Here's how the part is built. I have some questions about the finished solid (model axes, mm). A direction names the side the tool comes from. Coordinates: 2 decimals unless noted, no trailing zeros. Write each loop counter-clockwise with the first axis right and the second up, starting at its lowest first coordinate (ties: lowest second). Pieces come first, ordered by that corner, then holes.
from build123d import *

# Parameters (mm, degrees)
F1_DEPTH    = 5.5
F2_DEPTH    = 15
F3_T1_DEPTH = 64.5730638659
F3_T3_DEPTH = 54.5730638659


# Not quite as in the source:
# - a fillet or chamfer that OpenCascade refuses, or shapes differently, is made with other operations: its cross-section is extruded or revolved along the edge and cut away or added


with BuildPart() as f1:
    # F0 (on Right) → F1 (new body, symmetric)
    with BuildSketch(Plane.YZ):
        Polygon((-11, 0), (0, 0), (0, 5), (-11, 5), (-11, 11), (-15, 11), (-15, 0), align=None)
    extrude(amount=F1_DEPTH, both=True)

    # F0 (on Right) → F2 (join, symmetric)
    with BuildSketch(Plane.YZ):
        Polygon((-15, 15), (-15, 11), (-11, 11), (25, 11), (25, 15), align=None)
    extrude(amount=F2_DEPTH, both=True)

    # F3: chamfer of 4 x 4.7670143704 on 3 edges, made by hand

    # F3_s2 → F3_t1 (cut)
    with BuildSketch(Plane.XZ.offset(-37.2865319329)):
        Polygon((15, 10.2329856296), (11, 15), (15, 15), align=None)
        Polygon((-15, 10.2329856296), (-11, 15), (-15, 15), align=None)
    extrude(amount=F3_T1_DEPTH, mode=Mode.SUBTRACT)

    # F3_s4 → F3_t3 (cut)
    with BuildSketch(Plane.YZ.offset(-27.2865319329)):
        Polygon((21, 15), (25, 10.2329856296), (25, 15), align=None)
    extrude(amount=F3_T3_DEPTH, mode=Mode.SUBTRACT)


solid = f1.part
1. I want a section at A-A (y = -10.5). List the corners of the cut face in (x, z) for me, then the cut area to 3 significant figures.
2. I want a section at D-D (y = 3). List the corners of the cut face in (x, z) for me.
3. I want a section at C-C (z = 1.75). List the corners of the cut face in (x, y) for me, then the cut area to 3 significant figures.
4. I want a section at B-B (x = -1.5). List the corners of the cut face in (y, z) for me, then the cut area to 3 significant figures.
5. For pin 1 Ø3.5 at (y, z) = (-10, 4.5) entering from +X; pin 2 Ø3.5 at (y, z) = (-6.5, 4) entering from -X; pin 3 Ø3 at (x, z) = (1.5, 9) entering from +Y; pin 4 Ø1.5 at (y, z) = (2.5, 3.5) entering from -X, each with a flat end and sliding along its axis, tell me the tip position at first contact or that it passes through.
6. On a 3-axis mill with a long thin cutter (end or side, diameter ignored), from which of +Z, -Z, +X, -X, +Y, -Y can I reach the whole of each face in a straight line? I mean faces 5 (the face through (-5.5, -9, 3)), 6 (the face through (0, -8, 0)), 7 (the face through (5.5, -9, 3)). Say none if no direction works.
7. If I drill on line 1 (Z direction, x = -3.75, y = -10); line 2 (Z direction, x = 3.25, y = 12.5); line 3 (Y direction, x = 1, z = 10.75), over which ranges is the centre line in solid material (lowest first)?
8. Thinking about a two-plate mould opening in Z: for faces 1 (the face through (0, 0, 2)), 2 (the face through (0, -11, 8)), 3 (the face through (0, -5, 5)), 4 (the face through (-12.702, 4.954, 12.972)), which applies, pulls with the +Z half, pulls with the -Z half, needs draft (parallel to the pull), parting line crosses it, or undercut?
Response values:
1. outline: (-14.36, 11) - (14.36, 11) - (11, 15) - (-11, 15) - close; (-5.5, 0) - (5.5, 0) - (5.5, 5) - (-5.5, 5) - close
1. area: 156 mm2
2. outline: (-14.36, 11) - (14.36, 11) - (11, 15) - (-11, 15) - close
3. outline: (-5.5, -15) - (5.5, -15) - (5.5, 0) - (-5.5, 0) - close
3. area: 165 mm2
4. outline: (-15, 0) - (0, 0) - (0, 5) - (-11, 5) - (-11, 11) - (24.36, 11) - (21, 15) - (-15, 15) - close
4. area: 250 mm2
5. pin 1: stops at x = 5.5
5. pin 2: stops at x = -5.5
5. pin 3: stops at y = -11
5. pin 4: passes through
6. face 5: -Z, -X, +Y, -Y
6. face 6: -Z, +X, -X, +Y, -Y
6. face 7: -Z, +X, +Y, -Y
7. line 1: z = 0 to 5, 11 to 15
7. line 2: z = 11 to 15
7. line 3: y = -15 to -11
8. face 1: needs draft
8. face 2: undercut
8. face 3: undercut
8. face 4: pulls with the +Z half
